Work out the finished part from the listing and answer in its coordinate system (mm). A direction names the side the tool comes from. Give positions to 0.01 mm unless a question says otherwise; leave off trailing zeros. Loops run counter-clockwise (first coordinate to the right, second up) from the corner with the lowest first, then second, coordinate; pieces in that order, holes last.
from build123d import *

# Parameters (mm, degrees)
SKIZZE1_R                         = 60
SKIZZE1_R_2                       = 25.5
AUFSATZ_LINEAR_AUSTRAGEN1_DEPTH   = 2
AUFSATZ_LINEAR_AUSTRAGEN2_DEPTH   = 3.4
AUFSATZ_LINEAR_START              = 3.4
AUFSATZ_LINEAR_AUSTRAGEN3_DEPTH   = 1
DURCHGANGSLOCH_F_R_M41_AT_2_COUNT = 2
DURCHGANGSLOCH_F_R_M41_AT_2_PITCH = 16
VERRUNDUNG1_R                     = 3
KREISMUSTER3_COUNT                = 4
VERRUNDUNG1_OF_KREISMUSTER3_R     = 3
SCHNITT_LINEAR_AUSTRAGEN1_DEPTH   = 85.966817
KREISMUSTER4_COUNT                = 4


with BuildPart() as part:
    # Skizze1 → Aufsatz-Linear austragen1 (new body)
    with BuildSketch(Plane.XY):
        Circle(SKIZZE1_R)
        Circle(SKIZZE1_R_2, mode=Mode.SUBTRACT)
        with BuildLine():
            ThreePointArc((0, 35), (-24.748737, 24.748737), (-35, 0))
            ThreePointArc((-35, 0), (-31.5, -3.5), (-28, 0))
            ThreePointArc((-28, 0), (-19.79899, 19.79899), (0, 28))
            ThreePointArc((0, 28), (3.5, 31.5), (0, 35))
        make_face(mode=Mode.SUBTRACT)
        with BuildLine():
            ThreePointArc((35, 0), (24.748737, -24.748737), (0, -35))
            ThreePointArc((0, -35), (-3.5, -31.5), (0, -28))
            ThreePointArc((0, -28), (19.79899, -19.79899), (28, 0))
            ThreePointArc((28, 0), (31.5, 3.5), (35, 0))
        make_face(mode=Mode.SUBTRACT)
    extrude(amount=AUFSATZ_LINEAR_AUSTRAGEN1_DEPTH)

    # Skizze2 → Aufsatz-Linear austragen2 (add)
    with BuildSketch(Plane.XY.offset(2)):
        with BuildLine():
            Line((-15, 58.09475), (-15, 46.09475))
            Line((-15, 46.09475), (15, 46.09475))
            Line((15, 46.09475), (15, 58.09475))
            ThreePointArc((15, 58.09475), (0, 60), (-15, 58.09475))
        make_face()
        Polygon((-5.863804, 56.19475), (-10.136196, 56.19475), (-12.272392, 52.49475), (-10.136196, 48.79475), (-5.863804, 48.79475), (-3.727608, 52.49475), align=None, mode=Mode.SUBTRACT)
        Polygon((5.863804, 48.79475), (3.727608, 52.49475), (5.863804, 56.19475), (10.136196, 56.19475), (12.272392, 52.49475), (10.136196, 48.79475), align=None, mode=Mode.SUBTRACT)
    aufsatz_linear_austragen2 = extrude(amount=AUFSATZ_LINEAR_AUSTRAGEN2_DEPTH)

    # Skizze2_3 → Aufsatz-Linear austragen3 (add)
    with BuildSketch(Plane.XY.offset(2).offset(AUFSATZ_LINEAR_START)):
        with BuildLine():
            Line((-15, 58.09475), (-15, 46.09475))
            Line((-15, 46.09475), (15, 46.09475))
            Line((15, 46.09475), (15, 58.09475))
            ThreePointArc((15, 58.09475), (0, 60), (-15, 58.09475))
        make_face()
    aufsatz_linear_austragen3 = extrude(amount=AUFSATZ_LINEAR_AUSTRAGEN3_DEPTH)

    # Skizze4 → Durchgangsloch f_r M41 (revolve, cut)
    with BuildSketch(Plane(origin=(-8, 52.49475, 6.4), x_dir=(0, -1, 0), z_dir=(1, 0, 0))):
        Polygon((0, 0), (0, 65.742065), (2.4, 64.3), (2.4, 0), align=None)
    durchgangsloch_f_r_m41 = revolve(axis=Axis((-8, 52.49475, 12.75), (0, 0, -1)), mode=Mode.SUBTRACT)

    # Durchgangsloch f_r M41 at 2: Durchgangsloch f_r M41 ×2
    with Locations(*[(i * DURCHGANGSLOCH_F_R_M41_AT_2_PITCH, 0, 0) for i in range(1, DURCHGANGSLOCH_F_R_M41_AT_2_COUNT)]):
        add(durchgangsloch_f_r_m41, mode=Mode.SUBTRACT)

    # Verrundung1
    verrundung1_edges = [part.edges().sort_by_distance(p)[0] for p in [
        (-15, 46.09475, 4.2),
        (15, 46.09475, 4.2),
    ]]
    fillet(verrundung1_edges, radius=VERRUNDUNG1_R)

    # Kreismuster3: Aufsatz-Linear austragen2, Aufsatz-Linear austragen3, Durchgangsloch f_r M41 ×4 about axis
    kreismuster3_axis = Axis((0, 0, 0), (0, 0, 1))
    add([aufsatz_linear_austragen2.rotate(kreismuster3_axis, i * 360 / KREISMUSTER3_COUNT) for i in range(1, KREISMUSTER3_COUNT)])
    add([aufsatz_linear_austragen3.rotate(kreismuster3_axis, i * 360 / KREISMUSTER3_COUNT) for i in range(1, KREISMUSTER3_COUNT)])
    add([durchgangsloch_f_r_m41.rotate(kreismuster3_axis, i * 360 / KREISMUSTER3_COUNT) for i in range(1, KREISMUSTER3_COUNT)], mode=Mode.SUBTRACT)

    # Kreismuster3 copy 1 sketch → Kreismuster3 copy 1 (revolve, cut)
    with BuildSketch(Plane(origin=(-52.49475, 8, 6.4), x_dir=(1, 0, 0), z_dir=(0, 1, 0))):
        Polygon((0, 0), (0, 65.742065), (2.4, 64.3), (2.4, 0), align=None)
    revolve(axis=Axis((-52.49475, 8, 12.75), (0, 0, -1)), mode=Mode.SUBTRACT)

    # Kreismuster3 copy 2 sketch → Kreismuster3 copy 2 (revolve, cut)
    with BuildSketch(Plane(origin=(-8, -52.49475, 6.4), x_dir=(0, 1, 0), z_dir=(-1, 0, 0))):
        Polygon((0, 0), (0, 65.742065), (2.4, 64.3), (2.4, 0), align=None)
    revolve(axis=Axis((-8, -52.49475, 12.75), (0, 0, -1)), mode=Mode.SUBTRACT)

    # Kreismuster3 copy 3 sketch → Kreismuster3 copy 3 (revolve, cut)
    with BuildSketch(Plane(origin=(52.49475, -8, 6.4), x_dir=(-1, 0, 0), z_dir=(0, -1, 0))):
        Polygon((0, 0), (0, 65.742065), (2.4, 64.3), (2.4, 0), align=None)
    revolve(axis=Axis((52.49475, -8, 12.75), (0, 0, -1)), mode=Mode.SUBTRACT)

    # Verrundung1 of Kreismuster3
    verrundung1_of_kreismuster3_edges = [part.edges().sort_by_distance(p)[0] for p in [
        (-46.09475, -15, 4.2),
        (-46.09475, 15, 4.2),
        (15, -46.09475, 4.2),
        (-15, -46.09475, 4.2),
        (46.09475, 15, 4.2),
        (46.09475, -15, 4.2),
    ]]
    fillet(verrundung1_of_kreismuster3_edges, radius=VERRUNDUNG1_OF_KREISMUSTER3_R)

    # Skizze5 → Schnitt-Linear austragen1 (cut, through all)
    with BuildSketch(Plane.XY.offset(2)):
        with BuildLine():
            Line((58.09475, 15), (56.734019, 15))
            ThreePointArc((56.734019, 15), (27.223611, 27.223611), (15, 56.734019))
            Line((15, 56.734019), (15, 58.09475))
            ThreePointArc((15, 58.09475), (42.426407, 42.426407), (58.09475, 15))
        make_face()
    schnitt_linear_austragen1 = extrude(amount=-SCHNITT_LINEAR_AUSTRAGEN1_DEPTH, mode=Mode.SUBTRACT)

    # Kreismuster4: Schnitt-Linear austragen1 ×4 about axis
    kreismuster4_axis = Axis((0, 0, 0), (0, 0, 1))
    for i in range(1, KREISMUSTER4_COUNT):
        add(schnitt_linear_austragen1.rotate(kreismuster4_axis, i * 360 / KREISMUSTER4_COUNT), mode=Mode.SUBTRACT)


solid = part.part
Item 1: Find section A-A, the plane x = 31.5. Write down the section's boundary in (y, z).
Item 2: Consider line 1 (X direction, y = 49, z = 4); line 2 (Y direction, x = -8, z = 6.15); line 3 (Y direction, x = 51.5, z = 6). Determine where each line is inside the solid, lowest interval first.
Item 3: Find section D-D, the plane y = 8. Give the number of separate pieces and of enclosed holes in the cut face, plus the area to 3 significant figures.
Item 4: For faces 4 (the face through (8, 56.195, 4)), 5 (the face through (-50.2, 7.3, 1)), determine the directions among +Z, -Z, +X, -X, +Y, -Y from which every point of the face is accessible in a straight line to the end or side of a thin tool.
Item 5: Flat-ended cylindrical pins translate along their axes: pin 1 Ø2 at (x, z) = (41.5, 1) entering from +Y; pin 2 Ø3.5 at (y, z) = (-7.5, 3.5) entering from -X; pin 3 Ø2.5 at (x, z) = (7, 3) entering from +Y; pin 4 Ø8 at (x, y) = (-10, 51.5) entering from +Z. Find the tip coordinate at first contact, or state that the pin passes through.
Item 6: Determine the mould class of faces 1 (the face through (11.22, 50.67, 3.68)), 2 (the face through (-7.3, -50.2, 1)), 3 (the face through (-53, 0, 6.4)) for opening direction Y: released by +Y, released by -Y, zero draft, split by the parting line, or undercut.
Item 7: Find section C-C, the plane x = 18.5. Write down the section's boundary in (y, z).
Ans:
1. outline: (-23.49, 0) - (-15.26, 0) - (-15.26, 2) - (-23.49, 2) - close; (3.5, 0) - (23.49, 0) - (23.49, 2) - (3.5, 2) - close
2. line 1: x = -15 to -10.25, -5.75 to 5.75, 10.25 to 15
2. line 2: y = -59.46 to -54.89, -50.09 to -46.09, 46.09 to 50.09, 54.89 to 59.46
2. line 3: y = -15 to -10.18, -5.82 to 5.82, 10.18 to 15
3. separate pieces: 5
3. enclosed holes: 0
3. area: 165 mm2
4. face 4: none
4. face 5: +Z, -Z
5. pin 1: stops at y = 18.29
5. pin 2: stops at x = -59.72
5. pin 3: stops at y = 59.72
5. pin 4: stops at z = 6.4
6. face 1: undercut
6. face 2: undercut
6. face 3: zero draft
7. outline: (-40, 0) - (-29.71, 0) - (-29.71, 2) - (-40, 2) - close; (-21.02, 0) - (-17.55, 0) - (-17.55, 2) - (-21.02, 2) - close; (17.55, 0) - (40, 0) - (40, 2) - (17.55, 2) - close
